Geometry check sheet. Reference: the model listing, model coordinates, mm. A direction names the side the tool comes from. Round coordinates to 2 decimals unless told otherwise and drop trailing zeros. Order: outer loops, then holes, each group sorted by start corner. A loop starts at its lowest first (then second) coordinate and runs counter-clockwise, first axis right, second up. Notation, with made-up numbers: M 4,85.5 L 34,85.5 A23 cw 34,111.5 Z; hole C 47,13 d10. An arc over 180 degrees is marked long. Return JSON: item names as keys, results as strings. Group by question number.
```python
from build123d import *

# Parameters (mm, degrees)
BOSS_EXTRU_2_DEPTH = 5


with BuildPart() as part:
    # Esquisse2 → Boss.-Extru.2 (new body)
    with BuildSketch(Plane.XY):
        with BuildLine():
            Line((-440, 0), (-400, -69.282032303))
            ThreePointArc((-400, -69.282032303), (-387.855872826, -78.600548829), (-372.679491924, -76.602540378))
            Line((-372.679491924, -76.602540378), (-325.048094716, -49.102540378))
            Line((-325.048094716, -49.102540378), (-119.689110868, -49.102540378))
            ThreePointArc((-119.689110868, -49.102540378), (-102.368602792, -59.102540378), (-102.368602792, -79.102540378))
            Line((-102.368602792, -79.102540378), (-205.048094716, -256.948637287))
            Line((-205.048094716, -256.948637287), (-252.679491924, -284.448637287))
            ThreePointArc((-252.679491924, -284.448637287), (-261.99800845, -296.59276446), (-260, -311.769145362))
            Line((-260, -311.769145362), (-220, -381.051177665))
            Line((-220, -381.051177665), (-140, -381.051177665))
            ThreePointArc((-140, -381.051177665), (-125.857864376, -375.193313289), (-120, -361.051177665))
            Line((-120, -361.051177665), (-120, -306.051177665))
            Line((-120, -306.051177665), (-17.320508076, -128.205080757))
            ThreePointArc((-17.320508076, -128.205080757), (0, -118.205080757), (17.320508076, -128.205080757))
            Line((17.320508076, -128.205080757), (120, -306.051177665))
            Line((120, -306.051177665), (120, -361.051177665))
            ThreePointArc((120, -361.051177665), (125.857864376, -375.193313289), (140, -381.051177665))
            Line((140, -381.051177665), (220, -381.051177665))
            Line((220, -381.051177665), (260, -311.769145362))
            ThreePointArc((260, -311.769145362), (261.99800845, -296.59276446), (252.679491924, -284.448637287))
            Line((252.679491924, -284.448637287), (205.048094716, -256.948637287))
            Line((205.048094716, -256.948637287), (102.368602792, -79.102540378))
            ThreePointArc((102.368602792, -79.102540378), (102.368602792, -59.102540378), (119.689110868, -49.102540378))
            Line((119.689110868, -49.102540378), (325.048094716, -49.102540378))
            Line((325.048094716, -49.102540378), (372.679491924, -76.602540378))
            ThreePointArc((372.679491924, -76.602540378), (387.855872826, -78.600548829), (400, -69.282032303))
            Line((400, -69.282032303), (440, 0))
            Line((440, 0), (400, 69.282032303))
            ThreePointArc((400, 69.282032303), (387.855872826, 78.600548829), (372.679491924, 76.602540378))
            Line((372.679491924, 76.602540378), (325.048094716, 49.102540378))
            Line((325.048094716, 49.102540378), (119.689110868, 49.102540378))
            ThreePointArc((119.689110868, 49.102540378), (102.368602792, 59.102540378), (102.368602792, 79.102540378))
            Line((102.368602792, 79.102540378), (205.048094716, 256.948637287))
            Line((205.048094716, 256.948637287), (252.679491924, 284.448637287))
            ThreePointArc((252.679491924, 284.448637287), (261.99800845, 296.59276446), (260, 311.769145362))
            Line((260, 311.769145362), (220, 381.051177665))
            Line((220, 381.051177665), (140, 381.051177665))
            ThreePointArc((140, 381.051177665), (125.857864376, 375.193313289), (120, 361.051177665))
            Line((120, 361.051177665), (120, 306.051177665))
            Line((120, 306.051177665), (17.320508076, 128.205080757))
            ThreePointArc((17.320508076, 128.205080757), (0, 118.205080757), (-17.320508076, 128.205080757))
            Line((-17.320508076, 128.205080757), (-120, 306.051177665))
            Line((-120, 306.051177665), (-120, 361.051177665))
            ThreePointArc((-120, 361.051177665), (-125.857864376, 375.193313289), (-140, 381.051177665))
            Line((-140, 381.051177665), (-220, 381.051177665))
            Line((-220, 381.051177665), (-260, 311.769145362))
            ThreePointArc((-260, 311.769145362), (-261.99800845, 296.59276446), (-252.679491924, 284.448637287))
            Line((-252.679491924, 284.448637287), (-205.048094716, 256.948637287))
            Line((-205.048094716, 256.948637287), (-102.368602792, 79.102540378))
            ThreePointArc((-102.368602792, 79.102540378), (-102.368602792, 59.102540378), (-119.689110868, 49.102540378))
            Line((-119.689110868, 49.102540378), (-325.048094716, 49.102540378))
            Line((-325.048094716, 49.102540378), (-372.679491924, 76.602540378))
            ThreePointArc((-372.679491924, 76.602540378), (-387.855872826, 78.600548829), (-400, 69.282032303))
            Line((-400, 69.282032303), (-440, 0))
        make_face()
    extrude(amount=BOSS_EXTRU_2_DEPTH)


solid = part.part
```
Q1. Section check B-B on y = 223. Record the cut outline in (x, z).
Q2. Section check D-D on y = -97.5. Record the cut outline in (x, z).
Q3. Set-up check for faces 4 (the face through (228.53, 270.506, 2.465)), 5 (the face through (102.517, 58.85, 2.465)), 6 (the face through (348.53, -62.66, 2.46)): record each of +Z, -Z, +X, -X, +Y, -Y from which the full face is reachable in a straight line by a thin tool's end or side.
Q4. Section check A-A on x = -174. Record the cut outline in (y, z), plus the area to 3 significant figures.
Q5. Section check C-C on x = 285.5. Record the cut outline in (y, z).
Q6. Depth check by flat-ended pin: pin 1 Ø1.5 at (x, z) = (-63.5, 2.5) entering from -Y; pin 2 Ø1.5 at (y, z) = (57.5, 1.5) entering from -X; pin 3 Ø1.5 at (y, z) = (-333.5, 1.5) entering from -X. Enter the tip coordinate at first touch or a pass-through.
Q7. Release check for a two-part mould opening along Y. For faces 1 (the face through (-67.94, 215.88, 2.46)), 2 (the face through (-228.53, -270.506, 2.465)), 3 (the face through (-126.014, -375.348, 2.465)) record: +Y half, -Y half, draft (parallel to the pull), parting line (faces both ways), or undercut.
Q8. Material ranges on line 1 along Y through (x, z) = (-155.5, 2.95); line 2 along Y through (x, z) = (-154, 3.6); line 3 along Y through (x, z) = (324, 3.3), recorded low to high.
Geometry check:
{
 "1": {"outline": "M -185.45,0 L -72.05,0 L -72.05,5 L -185.45,5 Z; M 72.05,0 L 185.45,0 L 185.45,5 L 72.05,5 Z"},
 "2": {"outline": "M -112.99,0 L 112.99,0 L 112.99,5 L -112.99,5 Z"},
 "3": {"face 4": "+Z, -Z, +X", "face 5": "+Z, -Z", "face 6": "+Z, -Z, -Y"},
 "4": {"outline": "M -381.05,0 L -203.17,0 L -203.17,5 L -381.05,5 Z; M -49.1,0 L 49.1,0 L 49.1,5 L -49.1,5 Z; M 203.17,0 L 381.05,0 L 381.05,5 L 203.17,5 Z", "area": "2,270 mm^2"},
 "5": {"outline": "M -49.1,0 L 49.1,0 L 49.1,5 L -49.1,5 Z"},
 "6": {"pin 1": "stops at y = -209.49", "pin 2": "stops at x = -407.24", "pin 3": "stops at x = -247.89"},
 "7": {"face 1": "+Y half", "face 2": "undercut", "face 3": "-Y half"},
 "8": {"line 1": "y = -381.05 to -171.13, -49.1 to 49.1, 171.13 to 381.05", "line 2": "y = -381.05 to -168.53, -49.1 to 49.1, 168.53 to 381.05", "line 3": "y = -49.1 to 49.1"}
}
